Geometry: see drawing. Coordinates: mm, zero at the bounding-box minimum. Coordinates: 2 decimals unless noted, no trailing zeros. Loops run counter-clockwise (first coordinate to the right, second up) from the corner with the lowest first, then second, coordinate; pieces in that order, holes last. Notation, with made-up numbers: (72, 69.25) - (91, 69.25) arc R7 cw to (91, 79.25) - close; hole circle Ø2 at (59.5, 5). An arc over 180 degrees is marked (long way). Use a Markdown table: item, result. Add a question column.
1. Ray query, L1, parallel to Z at x = 42.5, y = 0.8; L2, parallel to X at y = 7.25, z = 26.5; L3, parallel to X at y = 10.75, z = 10.5. Return the intervals inside material, ascending. Write a range as [from, to].
2. Section query C-C on y = 5.5. Return the cut outline in (x, z).
3. Section query B-B on z = 3.5. Return the cut outline in (x, y) (3 decimals).
4. Draft query along X for the marked faces 1, 2, 3 and 4. Return one class per face: released by +X, released by -X, zero draft, split by the parting line, or undercut.
5. Contact query for flat-ended pins moving along their axis: P1, Ø12, axis at x = 18.5, z = 79.5, coming from the +Y side; P2, Ø4, axis at x = 42.5, z = 58.25, coming from the +Y side; P3, Ø5.5, axis at x = 42.5, z = 46.25, coming from the +Y side. Output: stop coordinate, or through.
6. Section query A-A on x = 66.5. Return the cut outline in (y, z), then the cut area to 3 significant figures.
7. Section query D-D on z = 58.25. Return the cut outline in (x, y).
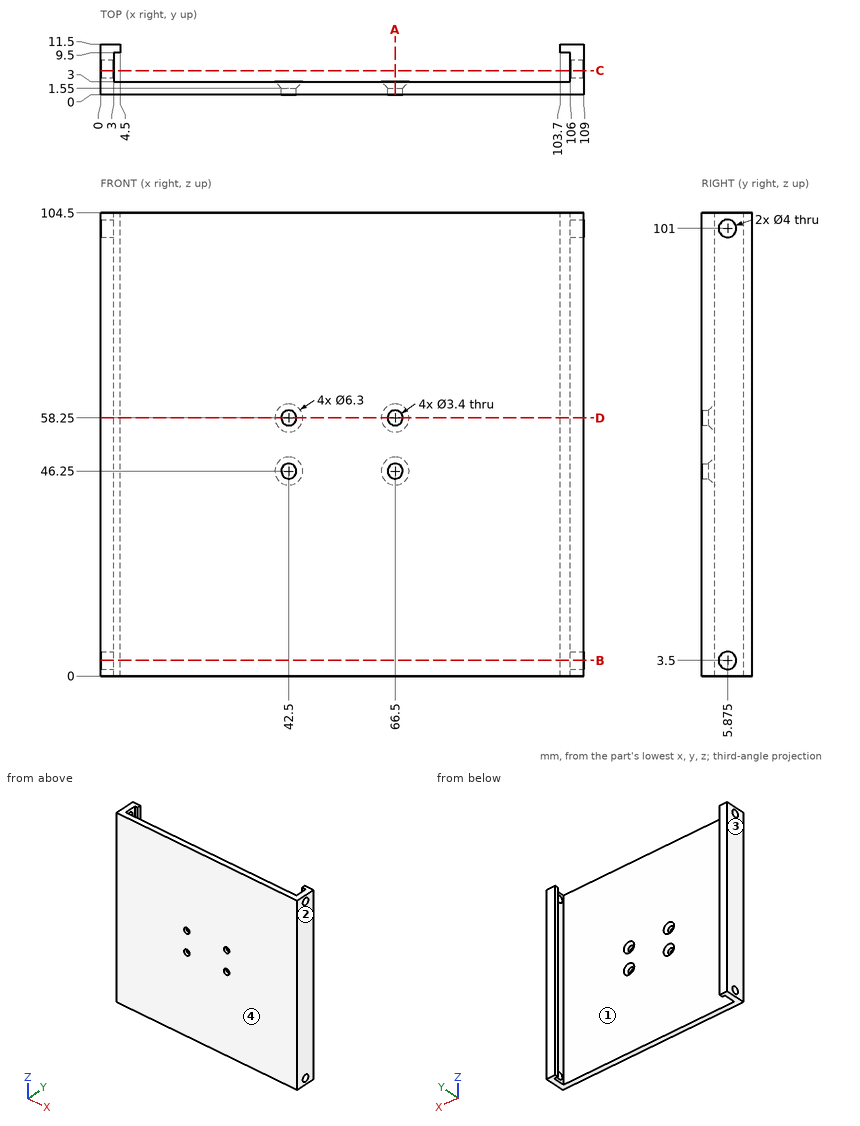
Resolved:
| question | item | result |
|---|---|---|
| 1 | L1 | [0, 44.55], [47.95, 56.55], [59.95, 104.5] |
| 1 | L2 | [0, 3], [106, 109] |
| 1 | L3 | [0, 4.5], [103.7, 109] |
| 2 | outline | (0, 0) - (3, 0) - (3, 1.54) - (0, 1.54) - close; (0, 5.46) - (3, 5.46) - (3, 99.04) - (0, 99.04) - close; (0, 102.96) - (3, 102.96) - (3, 104.5) - (0, 104.5) - close; (106, 0) - (109, 0) - (109, 1.54) - (106, 1.54) - close; (106, 5.46) - (109, 5.46) - (109, 99.04) - (106, 99.04) - close; (106, 102.96) - (109, 102.96) - (109, 104.5) - (106, 104.5) - close |
| 3 | outline | (0, 0) - (109, 0) - (109, 3.875) - (106, 3.875) - (106, 3) - (3, 3) - (3, 3.875) - (0, 3.875) - close; (0, 7.875) - (3, 7.875) - (3, 9.5) - (4.5, 9.5) - (4.5, 11.5) - (0, 11.5) - close; (103.7, 9.5) - (106, 9.5) - (106, 7.875) - (109, 7.875) - (109, 11.5) - (103.7, 11.5) - close |
| 4 | face 1 | undercut |
| 4 | face 2 | released by +X |
| 4 | face 3 | released by -X |
| 4 | face 4 | zero draft |
| 5 | P1 | y = 3 |
| 5 | P2 | y = 1.85 |
| 5 | P3 | y = 2.6 |
| 6 | outline | (0, 0) - (3, 0) - (3, 43.1) - (1.55, 44.55) - (0, 44.55) - close; (0, 47.95) - (1.55, 47.95) - (3, 49.4) - (3, 55.1) - (1.55, 56.55) - (0, 56.55) - close; (0, 59.95) - (1.55, 59.95) - (3, 61.4) - (3, 104.5) - (0, 104.5) - close |
| 6 | area | 289 mm² |
| 7 | outline | (0, 0) - (40.8, 0) - (40.8, 1.55) - (39.35, 3) - (3, 3) - (3, 9.5) - (4.5, 9.5) - (4.5, 11.5) - (0, 11.5) - close; (44.2, 0) - (64.8, 0) - (64.8, 1.55) - (63.35, 3) - (45.65, 3) - (44.2, 1.55) - close; (68.2, 0) - (109, 0) - (109, 11.5) - (103.7, 11.5) - (103.7, 9.5) - (106, 9.5) - (106, 3) - (69.65, 3) - (68.2, 1.55) - close |
